Design review of the part built by this model. Coordinates are the model's own, in mm. Give positions to 0.01 mm unless a question says otherwise; leave off trailing zeros. Loops run counter-clockwise (first coordinate to the right, second up) from the corner with the lowest first, then second, coordinate; pieces in that order, holes last. Notation, with made-up numbers: M 85,72.25 L 130,72.25 A24 ccw 130,84.25 Z; hole C 50,69 d10. An arc over 180 degrees is marked long. Answer as CSV lines item,"result".
Autodesk Inventor part; units mm, degrees
ref_plane "Work Plane1" through (13.2035, 0, 0) normal (0, 0, 1) x (-1, 0, 0)
ref_plane "YZ Plane" through (0, 0, 0) normal (1, 0, 0) x (0, 1, 0)
ref_plane "XZ Plane" through (0, 0, 0) normal (0, 1, 0) x (-1, 0, 0)
sketch "Sketch1" plane through (0, 0, 0) normal (1, 0, 0) x (0, 1, 0)
  line L0 (-4.6188, 0) -> (-2.3094, 4)
  line L1 (-2.3094, 4) -> (2.3094, 4)
  line L2 (2.3094, 4) -> (4.6188, 0)
  line L3 (4.6188, 0) -> (2.3094, -4)
  line L4 (2.3094, -4) -> (-2.3094, -4)
  line L5 (-2.3094, -4) -> (-4.6188, 0)
  point P0 (0, 0)
  point P1 (0, 0)
  dimension "d0" = 9.2376
extrude "Body" add sketch "Sketch1" along normal blind 5
sketch "Sketch2" plane through (0, 0, 0) normal (-1, 0, 0) x (0, 0, 1)
  line L0 (0, -6.4663) -> (0, 6.4663)
  line L1 (-5.6, 0) -> (5.6, 0)
  point P0 (0, 0)
hole "Thread" at (0, 0, 0) direction (1, 0, 0) diameter 4.134 end through all
chamfer "Chamfer1" distance 0.433 angle 30 1 edges at (0, 0, -2.067) measured on face at (0, -2.8764, -1.7247)
chamfer "Chamfer2" distance 0.433 angle 30 1 edges at (5, 0, -2.067) measured on face at (5, -2.8764, -1.7247)
sketch "Sketch3" plane through (0, 0, 0) normal (0, 0, 1) x (1, 0, 0)
  line L0 (0, 2.3094) -> (0, 4.6188)
  line L1 (0, 4.6188) -> (5, 4.6188)
  line L2 (5, 2.3094) -> (5, 4.6188)
  line L3 (-1.36, 0) -> (8.16, 0)
  line L4 (0.3573, 4.6188) -> (0, 4)
  line L5 (5, 4) -> (4.0192, 4)
  line L6 (4.0192, 4) -> (3.5, 4.6188)
  line L7 (13.2445, 4.6188) -> (17.2445, 2.3094) construction
  line L8 (17.2445, 2.3094) -> (17.2445, -2.3094) construction
  line L9 (17.2445, -2.3094) -> (13.2445, -4.6188) construction
  line L10 (13.2445, -4.6188) -> (9.2445, -2.3094) construction
  line L11 (9.2445, -2.3094) -> (9.2445, 2.3094) construction
  line L12 (9.2445, 2.3094) -> (13.2445, 4.6188) construction
  circle A0 centre (13.2445, 0) radius 4 construction
  line L13 (13.2445, 4) -> (5, 4) construction
  dimension "d3" = 30
  dimension "d5" = 8
  dimension "d8" = 40
  dimension "d9" = 3.5
  dimension "d43" = 8.2445
revolve "Chamfer3" cut sketch "Sketch3" angle 360 about axis through (-10, 0, 0) along (1, 0, 0)
ref_plane "Work Plane1" through (13.2035, 0, 0) normal (0, 0, 1) x (-1, 0, 0)
fillet "Fillet1" radius 0.3 1 edges at (5, -4, 0)
equation "\"d0\" = 1.1547 * SW"
equation "\"d3\" = ANG1"
equation "\"d5\" = SW0"
equation "\"d10\" = -0.5 * GD1 + 0.5 * NND"
equation "\"d39\" = -0.5 * GD1 + 0.5 * NND"
equation "\"d12\" = -0.5 * GD1 + 0.5 * NND"
equation "\"d40\" = -0.5 * GD1 + 0.5 * NND"
equation "\"ANG1\" = 30deg"
equation "\"ANG2\" = 60deg"
equation "\"NND\" = 5"
equation "\"KOH\" = 6.8"
equation "\"SW\" = 8"
equation "\"SW0\" = SW"
equation "\"SW1\" = 0.85 * SW"
equation "\"KOH1\" = 2.7"
equation "\"GUL\" = 0.541266 * PTC"
equation "\"THREADDIA\" = 5"
equation "\"TOA\" = 30deg"
equation "\"PTC\" = 0.8"
equation "\"E0\" = 1.155 * SW"
equation "\"GAL\" = 0.541266 * PTC"
properties part number "ParlocM5" material "Steel, Mild"
1. To check wall thickness, follow L1, parallel to Z at x = 2.95, y = 0; L2, parallel to Y at x = 3.8, z = 1.25; L3, parallel to Z at x = 2.3, y = 1.25. State the ranges of each line that lie inside material, in increasing order. Write a range as [from, to].
Answer block:
L1,"[-4, -2.07], [2.07, 4]"
L2,"[-3.9, -1.65], [1.65, 3.9]"
L3,"[-4, -1.65], [1.65, 4]"
2. We need section A-A, the plane x = 2.25. Write out the cut boundary in (y, z), plus the area to 3 significant figures.
Answer block:
outline,"M -4.62,0 L -2.31,-4 L 2.31,-4 L 4.62,0 L 2.31,4 L -2.31,4 Z; hole C 0,0 d4.13"
area,"42.0 mm²"
3. The part is to be moulded in two halves that separate along Z. For faces 1 (the conical face through (3.912, -2.071, 3.57)), 2 (the cylindrical face through (2.53, 1.26, -1.64)), 3 (the flat face through (2, 0, -4)), say which applies: pulls with the +Z half, pulls with the -Z half, needs draft (parallel to the pull), parting line crosses it, or undercut.
Answer block:
face 1,"pulls with the +Z half"
face 2,"undercut"
face 3,"pulls with the -Z half"
4. For P1, Ø2, axis at x = 3.5, z = 2, coming from the +Y side; P2, Ø2, axis at x = 3.5, z = 2.5, coming from the +Y side, all flat-tipped, find the tip position at first contact; note any pin that passes through.
Answer block:
P1,"y = 4.04"
P2,"y = 3.75"
